Part model, mm, in its own coordinate system. A direction names the side the tool comes from. Round coordinates to 2 decimals unless told otherwise and drop trailing zeros. Loops run counter-clockwise (first coordinate to the right, second up) from the corner with the lowest first, then second, coordinate; pieces in that order, holes last.
(1) Tool access for faces 1 (the face through (0, -24, 21.2)), 2 (the face through (23.8, -21, 7)): list every direction of +Z, -Z, +X, -X, +Y, -Y with a clear straight run to the whole face (end or side of a thin tool).
(2) Cut at D-D on z = 8. List the corners of the cut face in (x, y).
(3) Cut at B-B on z = 11.2. List the corners of the cut face in (x, y).
(4) Flat gauge pins, fed straight in: pin 1 (24.5 mm diameter, centred on x = -1.5, y = -3, fed in from +Z); pin 2 (10 mm diameter, centred on x = 14, z = 17.5, fed in from +Y). Where does each tip first touch, or does it go through?
(5) Cut at C-C on x = -16.5. List the corners of the cut face in (y, z), then the cut area to 3 significant figures.
(6) Cut at A-A on x = 0. List the corners of the cut face in (y, z).
(7) Mould opens along X. For faces 3 (the face through (25, -17, 6)), 4 (the face through (0, -23.8, 7)), 5 (the face through (0, 0, 0)), 6 (the face through (-25, -17, 6)) say: +X half, -X half, draft (parallel to the pull), parting line (faces both ways), or undercut.
(8) Probe probe 1 along Z at (x, y) = (0, -24.4); probe 2 along Z at (x, y) = (5, 22.5); probe 3 along Y at (x, z) = (23, 18.75). List the from-to ranges inside material, lowest first.
from build123d import *

# Parameters (mm, degrees)
SKETCH_W     = 50
SKETCH_H     = 50
PAD_DEPTH    = 1.2
SKETCH001_W  = 50
SKETCH001_H  = 1.2
PAD001_DEPTH = 20
PAD002_DEPTH = 1.2
PAD003_DEPTH = 1.2
SKETCH004_R  = 4
POCKET_DEPTH = 1.2


with BuildPart() as part:
    # Sketch → Pad (new body)
    with BuildSketch(Plane.XY):
        Rectangle(SKETCH_W, SKETCH_H)
    extrude(amount=PAD_DEPTH)

    # Sketch001 (on Face6 of Pad) → Pad001 (join)
    with BuildSketch(Plane.XY.offset(1.2)):
        with Locations((0, -24.4)):
            Rectangle(SKETCH001_W, SKETCH001_H)
    extrude(amount=PAD001_DEPTH)

    # Sketch002 (on Face7 of Pad001) → Pad002 (join)
    with BuildSketch(Plane(origin=(-25, 0, 0), x_dir=(0, -1, 0), z_dir=(-1, 0, 0))):
        Polygon((23.8, 21.2), (23.8, 1.2), (13.8, 1.2), align=None)
    extrude(amount=-PAD002_DEPTH)

    # Sketch003 (on Face1 of Pad002) → Pad003 (join)
    with BuildSketch(Plane.YZ.offset(25)):
        Polygon((-23.8, 21.2), (-23.8, 1.2), (-13.8, 1.2), align=None)
    extrude(amount=-PAD003_DEPTH)

    # Sketch004 (on Face9 of Pad003) → Pocket (cut)
    with BuildSketch(Plane.XZ.offset(25)):
        with Locations((0, 11.2)):
            Circle(SKETCH004_R)
    extrude(amount=-POCKET_DEPTH, mode=Mode.SUBTRACT)


solid = part.part
Final values:
1. face 1: +Z, +X, -X, +Y, -Y
1. face 2: +Z, +Y
2. outline: (-25, -25) - (-2.4, -25) - (-2.4, -23.8) - (-23.8, -23.8) - (-23.8, -17.2) - (-25, -17.2) - close; (2.4, -25) - (25, -25) - (25, -17.2) - (23.8, -17.2) - (23.8, -23.8) - (2.4, -23.8) - close
3. outline: (-25, -25) - (-4, -25) - (-4, -23.8) - (-23.8, -23.8) - (-23.8, -18.8) - (-25, -18.8) - close; (4, -25) - (25, -25) - (25, -18.8) - (23.8, -18.8) - (23.8, -23.8) - (4, -23.8) - close
4. pin 1: stops at z = 1.2
4. pin 2: stops at y = -23.8
5. outline: (-25, 0) - (25, 0) - (25, 1.2) - (-23.8, 1.2) - (-23.8, 21.2) - (-25, 21.2) - close
5. area: 84.0 mm2
6. outline: (-25, 0) - (25, 0) - (25, 1.2) - (-23.8, 1.2) - (-23.8, 7.2) - (-25, 7.2) - close; (-25, 15.2) - (-23.8, 15.2) - (-23.8, 21.2) - (-25, 21.2) - close
7. face 3: +X half
7. face 4: undercut
7. face 5: draft
7. face 6: -X half
8. probe 1: z = 0 to 7.2, 15.2 to 21.2
8. probe 2: z = 0 to 1.2
8. probe 3: y = -25 to -23.8
